Work out the finished part from the listing and answer in its coordinate system (mm). A direction names the side the tool comes from. Coordinates: 2 decimals unless noted, no trailing zeros. Order: outer loops, then holes, each group sorted by start corner. A loop starts at its lowest first (then second) coordinate and runs counter-clockwise, first axis right, second up. Notation, with made-up numbers: (49.5, 48.5) - (94.5, 48.5) arc R14 ccw to (94.5, 55.5) - close; hole circle Ø4 at (26.5, 52). An arc over 180 degrees is marked (long way). Answer as a JSON object with one key per item and string values. Group by question number.
1) Section B-B (y = 15) is taken. Give the vertices of the cut face in (x, z).
2) Section C-C (x = 8.5) is taken. Give the vertices of the cut face in (y, z).
3) A tool of negligible diameter and unlimited length cuts with its end or side. For faces 4 (the face through (21, 0, 30)), 5 (the face through (0, -16.5, 30)), 6 (the face through (0, -20, 5)), from which of +Z, -Z, +X, -X, +Y, -Y can it reach the whole face along a straight path? Write none if from no direction.
4) Section A-A (z = 26) is taken. Give the vertices of the cut face in (x, y).
5) Find the intervals of material crossed by line 1 along Y through (x, z) = (0, 3); line 2 along X through (y, z) = (-0.5, 29.5); line 3 along Y through (x, z) = (-6.5, 43), in increasing order.
6) The mould has two halves that part along X. Classify faces 1 (the face through (0.314, -5.303, 1.193)), 2 (the face through (-21, 0, 30)), 3 (the face through (-4.619, -1.915, 2.929)): released by +X, released by -X, zero draft, split by the parting line, or undercut.
7) Section D-D (y = -12) is taken. Give the vertices of the cut face in (x, z).
8) Each of these flat-tipped pins is pushed along its axis until it touches: P1, Ø3, axis at x = -13.5, y = 9, coming from the -Z side; P2, Ø13, axis at x = 0, y = 0, coming from the +Z side; P3, Ø12, axis at x = 1, z = 19, coming from the +Y side. Where does it stop, or does it pass through?
from build123d import *

# Parameters (mm, degrees)
SKETCH1_R               = 22.45
BOSS_EXTRUDE1_DEPTH     = 5
SKETCH2_R               = 5
CUT_EXTRUDE1_DEPTH      = 5
BOSS_EXTRUDE2_DEPTH     = 50
BOSS_EXTRUDE5_DEPTH     = 50
CUT_EXTRUDE3_DEPTH      = 64.505944604
CUT_EXTRUDE3_DEPTH_BACK = 64.505944604
CUT_EXTRUDE4_DEPTH      = 64.505944604
CUT_EXTRUDE4_DEPTH_BACK = 64.505944604
SKETCH7_R               = 0.5


with BuildPart() as part:
    # Sketch1 → Boss-Extrude1 (new body)
    with BuildSketch(Plane.XY):
        Circle(SKETCH1_R)
    extrude(amount=BOSS_EXTRUDE1_DEPTH)

    # Sketch2 → Cut-Extrude1 (cut)
    with BuildSketch(Plane(origin=(0, 0, 0), x_dir=(-1, 0, 0), z_dir=(0, 0, -1))):
        Circle(SKETCH2_R)
        with Locations((0, 15)):
            Circle(SKETCH2_R)
    extrude(amount=-CUT_EXTRUDE1_DEPTH, mode=Mode.SUBTRACT)

    # Sketch3 → Boss-Extrude2 (add)
    with BuildSketch(Plane.XY.offset(5)):
        with BuildLine():
            Line((-12.718195627, -18.5), (12.718195627, -18.5))
            ThreePointArc((12.718195627, -18.5), (14.006550731, -17.544772344), (15.223419458, -16.5))
            Line((15.223419458, -16.5), (-15.223419458, -16.5))
            ThreePointArc((-15.223419458, -16.5), (-14.006550731, -17.544772344), (-12.718195627, -18.5))
        make_face()
    extrude(amount=BOSS_EXTRUDE2_DEPTH)

    # Sketch5 → Boss-Extrude5 (add)
    with BuildSketch(Plane.XY.offset(5)):
        with BuildLine():
            Line((-15.223419458, -16.5), (-12.08108025, -16.5))
            ThreePointArc((-12.08108025, -16.5), (-12.994947259, -15.790308602), (-13.867212825, -15.030066815))
            ThreePointArc((-13.867212825, -15.030066815), (-18.732151535, -8.204206169), (-20.45, 0))
            Line((-20.45, 0), (-22.45, 0))
            ThreePointArc((-22.45, 0), (-20.564146795, -9.006573521), (-15.223419458, -16.5))
        make_face()
        with BuildLine():
            Line((20.45, 0), (22.45, 0))
            ThreePointArc((22.45, 0), (20.564146795, -9.006573521), (15.223419458, -16.5))
            Line((15.223419458, -16.5), (12.08108025, -16.5))
            ThreePointArc((12.08108025, -16.5), (12.994947259, -15.790308602), (13.867212825, -15.030066815))
            ThreePointArc((13.867212825, -15.030066815), (18.732151535, -8.204206169), (20.45, 0))
        make_face()
    extrude(amount=BOSS_EXTRUDE5_DEPTH)

    # Sketch6 → Cut-Extrude3 (cut, two sides: drawn at the far end of the back side and taken through both)
    with BuildSketch(Plane(origin=(0, 0, 0), x_dir=(1, 0, 0), z_dir=(0, 1, 0)).offset(-CUT_EXTRUDE3_DEPTH_BACK)):
        Polygon((-22.45, 0), (22.45, 0), (22.45, -2.35310929), align=None)
    extrude(amount=CUT_EXTRUDE3_DEPTH + CUT_EXTRUDE3_DEPTH_BACK, mode=Mode.SUBTRACT)

    # Sketch7 → Cut-Extrude4 (cut, two sides: drawn at the far end of the back side and taken through both)
    with BuildSketch(Plane(origin=(0, 0, 0), x_dir=(0, 0, -1), z_dir=(1, 0, 0)).offset(-CUT_EXTRUDE4_DEPTH_BACK)):
        with Locations((-50, -5)):
            Circle(SKETCH7_R)
        with Locations((-10, -5)):
            Circle(SKETCH7_R)
    extrude(amount=CUT_EXTRUDE4_DEPTH + CUT_EXTRUDE4_DEPTH_BACK, mode=Mode.SUBTRACT)


solid = part.part
Report:
{
 "1": {"outline": "(-16.7, 0.3) - (-5, 0.91) - (-5, 5) - (-16.7, 5) - close; (5, 1.44) - (16.7, 2.05) - (16.7, 5) - (5, 5) - close"},
 "2": {"outline": "(-20.78, 1.62) - (20.78, 1.62) - (20.78, 5) - (-16.5, 5) - (-16.5, 55) - (-18.5, 55) - (-18.5, 5) - (-20.78, 5) - close"},
 "3": {"face 4": "+Z, +X, -X, +Y", "face 5": "+Z, +Y", "face 6": "+Z, +X, -X, -Y"},
 "4": {"outline": "(-22.45, 0) arc R22.45 ccw to (-12.72, -18.5) - (12.72, -18.5) arc R22.45 ccw to (22.45, 0) - (20.45, 0) arc R20.45 cw to (12.08, -16.5) - (-12.08, -16.5) arc R20.45 cw to (-20.45, 0) - close"},
 "5": {"line 1": "y = -22.45 to -5, 5 to 10, 20 to 22.45", "line 2": "x = -22.44 to -20.44, 20.44 to 22.44", "line 3": "y = -18.5 to -16.5"},
 "6": {"face 1": "released by +X", "face 2": "zero draft", "face 3": "undercut"},
 "7": {"outline": "(-18.97, 0.18) - (18.97, 2.17) - (18.97, 55) - (16.56, 55) - (16.56, 5) - (-16.56, 5) - (-16.56, 55) - (-18.97, 55) - close"},
 "8": {"P1": "stops at z = 0.39", "P2": "stops at z = 5", "P3": "stops at y = -16.5"}
}
